Read the model definition and answer for the solid it produces. Units are mm, in the model's axes. A direction names the side the tool comes from. Round coordinates to 2 decimals unless told otherwise and drop trailing zeros. Loops run counter-clockwise (first coordinate to the right, second up) from the corner with the lowest first, then second, coordinate; pieces in that order, holes last. Notation, with made-up numbers: (39, 82) - (63, 82) arc R22 cw to (63, 107) - close; hole circle Ø11 at (-40, 26.5). An arc over 180 degrees is marked (long way). Answer as CSV lines item,"result".
```python
from build123d import *

# Parameters (mm, degrees)
BASE_FLANGE1_DEPTH      = 1.5
CUT_EXTRUDE1_DEPTH      = 11.017484714
CUT_EXTRUDE1_DEPTH_BACK = 11.017484714
SKETCH6_W               = 0.75
SKETCH6_H               = 3.25
FILLET1_R               = 0.3
FILLET2_R               = 0.3


# Sheet-metal steps are written as plain solids
with BuildPart() as part:
    # Sketch1 → Base-Flange1 (new, symmetric)
    with BuildSketch(Plane.XY):
        with BuildLine():
            Line((8.1, 0), (6.5, 0))
            ThreePointArc((6.5, 0), (6.217157288, -0.117157288), (6.1, -0.4))
            Line((6.1, -0.4), (6.1, -5.3))
            ThreePointArc((6.1, -5.3), (6.041421356, -5.441421356), (5.9, -5.5))
            Line((5.9, -5.5), (-5.9, -5.5))
            ThreePointArc((-5.9, -5.5), (-6.041421356, -5.441421356), (-6.1, -5.3))
            Line((-6.1, -5.3), (-6.1, -0.4))
            ThreePointArc((-6.1, -0.4), (-6.217157288, -0.117157288), (-6.5, 0))
            Line((-6.5, 0), (-8.1, 0))
            Line((-8.1, 0), (-8.1, -0.2))
            Line((-8.1, -0.2), (-6.5, -0.2))
            ThreePointArc((-6.5, -0.2), (-6.358578644, -0.258578644), (-6.3, -0.4))
            Line((-6.3, -0.4), (-6.3, -5.3))
            ThreePointArc((-6.3, -5.3), (-6.182842712, -5.582842712), (-5.9, -5.7))
            Line((-5.9, -5.7), (5.9, -5.7))
            ThreePointArc((5.9, -5.7), (6.182842712, -5.582842712), (6.3, -5.3))
            Line((6.3, -5.3), (6.3, -0.4))
            ThreePointArc((6.3, -0.4), (6.358578644, -0.258578644), (6.5, -0.2))
            Line((6.5, -0.2), (8.1, -0.2))
            Line((8.1, -0.2), (8.1, 0))
        make_face()
    extrude(amount=BASE_FLANGE1_DEPTH, both=True)

    # Sketch6 → Cut-Extrude1 (cut, two sides: drawn at the far end of the back side and taken through both)
    with BuildSketch(Plane(origin=(0, 0, 0), x_dir=(0, 0, -1), z_dir=(1, 0, 0)).offset(-CUT_EXTRUDE1_DEPTH_BACK)):
        with Locations((1.125, 0.875)):
            Rectangle(SKETCH6_W, SKETCH6_H)
        with Locations((-1.125, 0.875)):
            Rectangle(SKETCH6_W, SKETCH6_H)
    extrude(amount=CUT_EXTRUDE1_DEPTH + CUT_EXTRUDE1_DEPTH_BACK, mode=Mode.SUBTRACT)

    # Fillet1
    fillet1_edges = [part.edges().sort_by_distance(p)[0] for p in [
        (6.2, -0.75, -1.5),
        (-6.2, -0.75, -1.5),
        (6.2, -0.75, -0.75),
        (-6.2, -0.75, -0.75),
        (6.2, -0.75, 1.5),
        (-6.2, -0.75, 1.5),
        (6.2, -0.75, 0.75),
        (-6.2, -0.75, 0.75),
    ]]
    fillet(fillet1_edges, radius=FILLET1_R)

    # Fillet2
    fillet2_edges = [part.edges().sort_by_distance(p)[0] for p in [
        (-8.1, -0.1, -0.75),
        (8.1, -0.1, -0.75),
        (8.1, -0.1, 0.75),
        (-8.1, -0.1, 0.75),
    ]]
    fillet(fillet2_edges, radius=FILLET2_R)


solid = part.part
```
1) A tool of negligible diameter and unlimited length cuts with its end or side. For faces 1 (the face through (-7, -0.2, 0)), 2 (the face through (-7, 0, 0)), 3 (the face through (6.3, -3, 0)), 4 (the face through (-6.1, -3, 0)), from which of +Z, -Z, +X, -X, +Y, -Y can it reach the whole face along a straight path? Write none if from no direction.
Entries:
face 1,"+Z, -Z, -X, -Y"
face 2,"+Z, -Z, +X, -X, +Y"
face 3,"+Z, -Z, +X, -Y"
face 4,"+Z, -Z, +Y"
2) A cutting plane is placed at C-C, the plane y = -0.6. Determine the outline of the cut face in (x, z), plus the area to 3 significant figures.
Entries:
outline,"(-6.3, -0.79) - (-6.1, -0.79) - (-6.1, 0.79) - (-6.3, 0.79) - close; (6.1, -0.79) - (6.3, -0.79) - (6.3, 0.79) - (6.1, 0.79) - close"
area,"0.632 mm^2"
3) Find the intervals of material crossed by line 1 (X direction, y = -4.1, z = 0.25); line 2 (Y direction, x = 5.5, z = 1.1); line 3 (Y direction, x = -7.5, z = 0.05), in increasing order.
Entries:
line 1,"x = -6.3 to -6.1, 6.1 to 6.3"
line 2,"y = -5.7 to -5.5"
line 3,"y = -0.2 to 0"
4) A cutting plane is placed at D-D, the plane x = -3. Determine the outline of the cut face in (y, z), plus the area to 3 significant figures.
Entries:
outline,"(-5.7, -1.5) - (-5.5, -1.5) - (-5.5, 1.5) - (-5.7, 1.5) - close"
area,"0.600 mm^2"
5) A cutting plane is placed at A-A, the plane y = -3.45. Determine the outline of the cut face in (x, z).
Entries:
outline,"(-6.3, -1.5) - (-6.1, -1.5) - (-6.1, 1.5) - (-6.3, 1.5) - close; (6.1, -1.5) - (6.3, -1.5) - (6.3, 1.5) - (6.1, 1.5) - close"
6) Each of these flat-tipped pins is pushed along its axis until it touches: P1, Ø0.9, axis at y = -3.5, z = 0.5, coming from the -X side; P2, Ø1.6, axis at x = -7.5, z = 0, coming from the -Y side; P3, Ø1.5, axis at y = -3, z = 0.5, coming from the +X side. Where does it stop, or does it pass through?
Entries:
P1,"stops at x = -6.3"
P2,"stops at y = -0.2"
P3,"stops at x = 6.3"
7) A cutting plane is placed at B-B, the plane z = 0.2. Determine the outline of the cut face in (x, y), plus the area to 3 significant figures.
Entries:
outline,"(-8.1, -0.2) - (-6.5, -0.2) arc R0.2 cw to (-6.3, -0.4) - (-6.3, -5.3) arc R0.4 ccw to (-5.9, -5.7) - (5.9, -5.7) arc R0.4 ccw to (6.3, -5.3) - (6.3, -0.4) arc R0.2 cw to (6.5, -0.2) - (8.1, -0.2) - (8.1, 0) - (6.5, 0) arc R0.4 ccw to (6.1, -0.4) - (6.1, -5.3) arc R0.2 cw to (5.9, -5.5) - (-5.9, -5.5) arc R0.2 cw to (-6.1, -5.3) - (-6.1, -0.4) arc R0.4 ccw to (-6.5, 0) - (-8.1, 0) - close"
area,"5.34 mm^2"
8) The mould has two halves that part along X. Classify faces 5 (the face through (7, -0.2, 0)), 6 (the face through (-6.3, -3, 0)), 7 (the face through (6.1, -3, 0)): pulls with the +X half, pulls with the -X half, needs draft (parallel to the pull), parting line crosses it, or undercut.
Entries:
face 5,"needs draft"
face 6,"pulls with the -X half"
face 7,"undercut"
